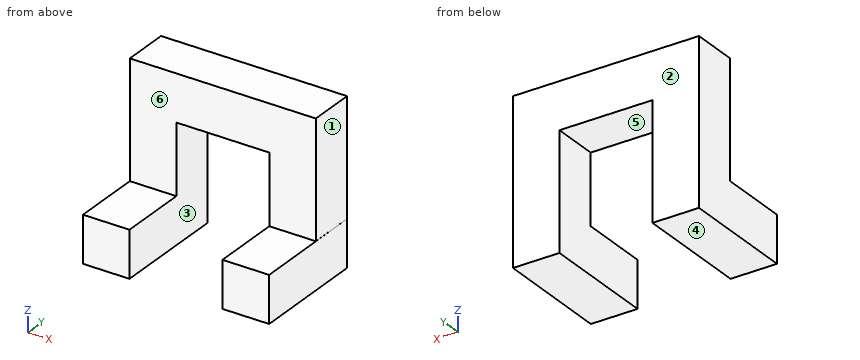
from build123d import *

# Parameters (mm, degrees)
F1_DEPTH = 50.8
F2_W     = 50.8
F2_H     = 127
F3_DEPTH = 50.8
F5_DEPTH = 50.8


with BuildPart() as f1:
    # F0 (on Front) → F1 (new body)
    with BuildSketch(Plane.XZ):
        Polygon((-98.19336, 70.319961), (-98.19336, -56.680039), (-47.39336, -56.680039), (-47.39336, 19.519961), (54.20664, 19.519961), (54.20664, -56.680039), (105.00664, -56.680039), (105.00664, 70.319961), align=None)
    extrude(amount=F1_DEPTH)

    # F2 (on face) → F3 (join)
    with BuildSketch(Plane(origin=(0, 0, -56.680039), x_dir=(1, 0, 0), z_dir=(0, 0, -1))):
        with Locations((-72.79336, 63.5)):
            Rectangle(F2_W, F2_H)
    extrude(amount=F3_DEPTH)

    # F4 (on face) → F5 (join)
    with BuildSketch(Plane(origin=(0, 0, -56.680039), x_dir=(1, 0, 0), z_dir=(0, 0, -1))):
        Polygon((54.20664, 126.999759), (54.20664, 0), (105.00664, 0), (105.254231, 126.999759), align=None)
    extrude(amount=F5_DEPTH)


solid = f1.part
Build history of the part. All positions in model axes, mm. Face numbers are marked on the shaded views. A direction names the side the tool comes from. Give positions to 0.01 mm unless a question says otherwise; leave off trailing zeros. Loops run counter-clockwise (first coordinate to the right, second up) from the corner with the lowest first, then second, coordinate; pieces in that order, holes last. Notation, with made-up numbers: (1, 50.25) -> (6, 50.25) arc R21 ccw to (6, 69.25) -> close; hole circle Ø9 at (21.25, 33.5). An arc over 180 degrees is marked (long way). Answer in a Markdown table with one row per item.
Item 1: Flat gauge pin, fed straight in: P1, Ø1.5, axis at x = -47.5, z = 6.5, coming from the -Y side. Where does the tip first touch, or does it go through?
Findings below:
| item | result |
|---|---|
| P1 | stops at y = -50.8 |
Item 2: Mould opens along X. For the marked faces 1, 2 and 3 say: pulls with the +X half, pulls with the -X half, needs draft (parallel to the pull), parting line crosses it, or undercut.
Findings below:
| item | result |
|---|---|
| face 1 | pulls with the +X half |
| face 2 | needs draft |
| face 3 | undercut |
Item 3: Tool access for the marked faces 4, 5 and 6: list every direction of +Z, -Z, +X, -X, +Y, -Y with a clear straight run to the whole face (end or side of a thin tool).
Findings below:
| item | result |
|---|---|
| face 4 | -Z, +X, -X, +Y, -Y |
| face 5 | -Z, +Y, -Y |
| face 6 | +Z, +X, -X, -Y |
Item 4: Slice it at A-A on z = -80. Write the cut outline in (x, y).
Findings below:
| item | result |
|---|---|
| outline | (-98.19, -127) -> (-47.39, -127) -> (-47.39, 0) -> (-98.19, 0) -> close; (54.21, -127) -> (105.25, -127) -> (105.01, 0) -> (54.21, 0) -> close |
Item 5: Slice it at B-B on y = -81. Write the cut outline in (x, z), plus the area to 3 significant figures.
Findings below:
| item | result |
|---|---|
| outline | (-98.19, -107.48) -> (-47.39, -107.48) -> (-47.39, -56.68) -> (-98.19, -56.68) -> close; (54.21, -107.48) -> (105.16, -107.48) -> (105.16, -56.68) -> (54.21, -56.68) -> close |
| area | 5,170 mm² |
Item 6: Probe line 1 along X through (y, z) = (-12, -72.5); line 2 along X through (y, z) = (-23, -73); line 3 along Z through (x, y) = (26.5, -35.5). List the from-to ranges inside material, lowest first. Write a range as [from, to].
Findings below:
| item | result |
|---|---|
| line 1 | x = [-98.19, -47.39], [54.21, 105.03] |
| line 2 | x = [-98.19, -47.39], [54.21, 105.05] |
| line 3 | z = [19.52, 70.32] |
Item 7: Slice it at C-C on x = 7.5. Write the cut outline in (y, z), plus the area to 3 significant figures.
Findings below:
| item | result |
|---|---|
| outline | (-50.8, 19.52) -> (0, 19.52) -> (0, 70.32) -> (-50.8, 70.32) -> close |
| area | 2,580 mm² |
